Verification items for the finished model (mm, model axes). A direction names the side the tool comes from. Round coordinates to 2 decimals unless told otherwise and drop trailing zeros. Write each loop counter-clockwise with the first axis right and the second up, starting at its lowest first coordinate (ties: lowest second). Pieces come first, ordered by that corner, then holes. Notation, with made-up numbers: M 80,72 L 114,72 A20 ccw 114,102 Z; hole C 59,83.25 d9. An arc over 180 degrees is marked long. One line per item, written item: value. Start each with the question number.
Item 1: Thickness scan on probe 1 along X at (y, z) = (-18, 18) (3 decimals); probe 2 along X at (y, z) = (-45.5, 3.5) (3 decimals); probe 3 along Y at (x, z) = (47, 54). Record the ranges inside material, lowest first. Write a range as from..to.
Item 2: Gauge pin test, flat ends, axial feed: pin 1 (4 mm diameter, centred on x = 54.5, y = -11.5, fed in from +Z); pin 2 (5 mm diameter, centred on y = -15.5, z = 19, fed in from -X) (3 decimals); pin 3 (11 mm diameter, centred on y = -13.5, z = 13.5, fed in from +X) (3 decimals). Record the tip position at first contact, or that the pin passes through.
Item 3: Section check C-C, the plane y = -43. Record the cut outline in (x, z) (3 decimals), then the cut area to 3 significant figures.
Item 4: Section check A-A, the plane z = 0. Record the cut outline in (x, y) (3 decimals).
Item 5: Draft check along X on faces 6 (the face through (45.8, -0.4, 38.1)), 7 (the face through (41.275, -1, 4)), 8 (the face through (-4, -7.938, 30)). Enter one of: +X half, -X half, draft (parallel to the pull), parting line (faces both ways), or undercut.
Item 6: Section check B-B, the plane x = 75.5. Record the cut outline in (y, z) (3 decimals).
Item 7: Tool access check on faces 1 (the face through (60, 2, 61.925)), 2 (the face through (-4, 7.938, 30)), 3 (the face through (22.225, -17, 18)), 4 (the face through (46, -25.4, 42)), 5 (the face through (46, 25.4, 42)). Record the directions out of +Z, -Z, +X, -X, +Y, -Y that give a thin tool (end or side, any length) a straight path to the whole face; none if there is none.
from build123d import *

# Parameters (mm, degrees)
F1_DEPTH = 63.5
F2_DEPTH = 25.4
F3_DEPTH = 7.9375
F0_W     = 25.4
F0_H     = 19.05
F4_DEPTH = 25.4
F6_R     = 6.35


with BuildPart() as f1:
    # F0 (on Front) → F1 (new body, symmetric)
    with BuildSketch(Plane.XZ):
        Polygon((22.225, 9.525), (-41.275, 9.525), (-41.275, -9.525), (41.275, -9.525), (41.275, 9.525), align=None)
    extrude(amount=F1_DEPTH, both=True)

    # F0 (on Front) → F2 (join, symmetric)
    with BuildSketch(Plane.XZ):
        with BuildLine():
            Line((22.225, 27.0002), (22.225, 9.525))
            Line((22.225, 9.525), (41.275, 9.525))
            Line((41.275, 9.525), (41.275, 27.0002))
            ThreePointArc((41.275, 27.0002), (45.9246798487, 38.2255201513), (57.15, 42.8752))
            Line((57.15, 42.8752), (60.325, 42.8752))
            Line((60.325, 42.8752), (60.325, 61.9252))
            Line((60.325, 61.9252), (57.15, 61.9252))
            add(Edge.make_bspline(
                [(52.1673264767, 61.5679391445), (53.8333829915, 61.7094866202), (55.4951364751, 61.8287124743), (57.15, 61.9252)],
                knots=[107.5205143307, 107.5205143307, 107.5205143307, 107.5205143307, 111.5045361635, 111.5045361635, 111.5045361635, 111.5045361635], degree=3))
            ThreePointArc((52.1673264767, 61.5679391445), (30.7513684275, 49.8665043822), (22.225, 27.0002))
        make_face()
    extrude(amount=F2_DEPTH, both=True)

    # F0 (on Front) → F3 (join, symmetric)
    with BuildSketch(Plane.XZ):
        with BuildLine():
            add(Edge.make_bspline(
                [(-41.275, 9.525), (-40.8936231026, 37.6698712219), (7.2039048673, 57.7478653509), (52.1673264767, 61.5679391445)],
                knots=[0, 0, 0, 0, 107.5205143307, 107.5205143307, 107.5205143307, 107.5205143307], degree=3))
            Line((-41.275, 9.525), (22.225, 9.525))
            Line((22.225, 9.525), (22.225, 27.0002))
            ThreePointArc((22.225, 27.0002), (30.7513684275, 49.8665043822), (52.1673264767, 61.5679391445))
        make_face()
    extrude(amount=F3_DEPTH, both=True)

    # F0 (on Front) → F4 (join, symmetric)
    with BuildSketch(Plane.XZ):
        with Locations((73.025, 52.4002)):
            Rectangle(F0_W, F0_H)
    extrude(amount=F4_DEPTH, both=True)

    # F0 (on Front) → F5 (revolve)
    with BuildSketch(Plane.XZ):
        Polygon((85.725, 66.675), (85.725, 61.9252), (85.725, 42.8752), (85.725, 38.1), (111.125, 38.1), (111.125, 66.675), align=None)
    revolve(axis=Axis((85.725, 0, 52.3875), (0, 0, 1)))

    # F6
    f6_edges = [f1.edges().sort_by_distance(p)[0] for p in [
        (-41.275, -63.5, 0),
        (41.275, -63.5, 0),
        (41.275, 63.5, 0),
        (-41.275, 63.5, 0),
    ]]
    fillet(f6_edges, radius=F6_R)


solid = f1.part
Response values:
1. probe 1: x = 22.225..41.275
1. probe 2: x = -41.275..41.275
1. probe 3: y = -25.4..25.4
2. pin 1: stops at z = 61.89
2. pin 2: stops at x = 22.225
2. pin 3: stops at x = 41.275
3. outline: M -41.275,-9.525 L 41.275,-9.525 L 41.275,9.525 L -41.275,9.525 Z
3. area: 1,570 mm2
4. outline: M -41.275,-57.15 A6.35 ccw -34.925,-63.5 L 34.925,-63.5 A6.35 ccw 41.275,-57.15 L 41.275,57.15 A6.35 ccw 34.925,63.5 L -34.925,63.5 A6.35 ccw -41.275,57.15 Z
5. face 6: undercut
5. face 7: +X half
5. face 8: draft
6. outline: M -25.4,42.875 L -23.251,42.875 L -23.251,38.1 L 23.251,38.1 L 23.251,42.875 L 25.4,42.875 L 25.4,61.925 L 23.251,61.925 L 23.251,66.675 L -23.251,66.675 L -23.251,61.925 L -25.4,61.925 Z
7. face 1: +Z, -X
7. face 2: +Z, -X, +Y
7. face 3: +Z, -X, -Y
7. face 4: +Z, +X, -X, -Y
7. face 5: +Z, +X, -X, +Y
